```python
from build123d import *

# Parameters (mm, degrees)
SKETCH1_R        = 8
EXTRUSION1_DEPTH = 400
SKETCH2_R        = 8
EXTRUSION2_DEPTH = 50
EXTRUSION3_START = 50
SKETCH3_R        = 8
EXTRUSION3_DEPTH = 50
SKETCH4_R        = 8
SKETCH4_R_2      = 6
THREAD1_DEPTH    = 14
SKETCH5_R        = 8
SKETCH5_R_2      = 6.05
EXTRUSION5_DEPTH = 25
SKETCH6_R        = 5
EXTRUSION6_DEPTH = 15
EXTRUSION7_START = -27.101
SKETCH7_R        = 8
EXTRUSION7_DEPTH = 27.101
EXTRUSION8_START = 12
SKETCH8_R        = 5
EXTRUSION8_DEPTH = 12


with BuildPart() as part:
    # Sketch1 → Extrusion1 (new body)
    with BuildSketch(Plane(origin=(0, 0, 0), x_dir=(-1, 0, 0), z_dir=(0, 1, 0))):
        with Locations(Location((0, 0, 0), (0, 0, 90))):
            Circle(SKETCH1_R)
    extrude(amount=EXTRUSION1_DEPTH)

    # Sketch2 → Extrusion2 (cut)
    with BuildSketch(Plane.XZ):
        with Locations(Location((0, 0, 0), (0, 0, 270))):
            Circle(SKETCH2_R)
    extrude(amount=-EXTRUSION2_DEPTH, mode=Mode.SUBTRACT)

    # Sketch3 → Extrusion3 (add)
    with BuildSketch(Plane.XZ.offset(-50).offset(EXTRUSION3_START)):
        with Locations(Location((0, 0, 0), (0, 0, 270))):
            Circle(SKETCH3_R)
    extrude(amount=-EXTRUSION3_DEPTH)

    # Sketch4 → Thread1 (cut)
    with BuildSketch(Plane.XZ):
        with Locations(Location((0, 0, 0), (0, 0, 270))):
            Circle(SKETCH4_R)
        with Locations(Location((0, 0, 0), (0, 0, 270))):
            Circle(SKETCH4_R_2, mode=Mode.SUBTRACT)
    extrude(amount=-THREAD1_DEPTH, mode=Mode.SUBTRACT)

    # Sketch5 → Extrusion5 (cut)
    with BuildSketch(Plane.XZ.offset(-14)):
        with Locations(Location((0, 0, 0), (0, 0, 270))):
            Circle(SKETCH5_R)
        with Locations(Location((0, 0, 0), (0, 0, 270))):
            Circle(SKETCH5_R_2, mode=Mode.SUBTRACT)
    extrude(amount=-EXTRUSION5_DEPTH, mode=Mode.SUBTRACT)

    # Sketch6 → Extrusion6 (add)
    with BuildSketch(Plane.XZ):
        with Locations(Location((0, 0, 0), (0, 0, 270))):
            Circle(SKETCH6_R)
    extrude(amount=EXTRUSION6_DEPTH)

    # Sketch7 → Extrusion7 (cut)
    with BuildSketch(Plane(origin=(0, 400, 0), x_dir=(-1, 0, 0), z_dir=(0, 1, 0)).offset(EXTRUSION7_START)):
        with Locations(Location((0, 0, 0), (0, 0, 270))):
            Circle(SKETCH7_R)
    extrude(amount=EXTRUSION7_DEPTH, mode=Mode.SUBTRACT)

    # Sketch8 → Extrusion8 (add)
    with BuildSketch(Plane(origin=(0, 372.899, 0), x_dir=(-1, 0, 0), z_dir=(0, 1, 0)).offset(EXTRUSION8_START)):
        with Locations(Location((0, 0, 0), (0, 0, 270))):
            Circle(SKETCH8_R)
    extrude(amount=-EXTRUSION8_DEPTH)


solid = part.part
```
Check sheet for the modelled part. Datum: model origin and axes. Units: mm. A direction names the side the tool comes from. Coordinates: 2 decimals unless noted, no trailing zeros. Order: outer loops, then holes, each group sorted by start corner. A loop starts at its lowest first (then second) coordinate and runs counter-clockwise, first axis right, second up. Notation, with made-up numbers: (34, 64) -> (62, 64) arc R20 ccw to (62, 77) -> close; hole circle Ø4 at (-6, 62.25). An arc over 180 degrees is marked (long way). Write each question's results on one line, items separated by ' | '. Start each with the question number.
1) Depth check by flat-ended pin: pin 1 (1 mm diameter, centred on y = 310.5, z = -6.5, fed in from +X); pin 2 (3 mm diameter, centred on x = 6, z = 4.5, fed in from +Y); pin 3 (2 mm diameter, centred on x = -3.5, y = 45, fed in from +Z); pin 4 (1.5 mm diameter, centred on x = 2.5, z = -4.5, fed in from -Y). Enter the tip coordinate at first touch or a pass-through.
2) Section check C-C (y = 67.5). Enter the section's corners in (x, z).
3) Material ranges on line 1 along X through (y, z) = (357, 0.5); line 2 along Z through (x, y) = (0.75, 297); line 3 along Y through (x, z) = (-1.75, -7), recorded low to high.
4) Set-up check for faces 1 (the face through (0, 384.899, 0)), 2 (the face through (4, 0, 4)), 3 (the face through (5.2, 372.899, 0.1)): record each of +Z, -Z, +X, -X, +Y, -Y from which the full face is reachable in a straight line by a thin tool's end or side.
5) Section check A-A (x = 0). Enter the section's corners in (y, z), and give its area (3 significant figures).
6) Section check B-B (z = 0). Enter the section's corners in (x, y).
Checked values:
1) pin 1: x = 5.29 | pin 2: y = 372.9 | pin 3: z = 7.6 | pin 4: y = -15
2) outline: circle Ø16 at (0, 0)
3) line 1: -7.98 to 7.98 | line 2: -7.96 to 7.96 | line 3: 39 to 372.9
4) face 1: +Z, -Z, +X, -X, +Y | face 2: -Y | face 3: +Y
5) outline: (-15, -5) -> (0, -5) -> (0, -6) -> (14, -6) -> (14, -6.05) -> (39, -6.05) -> (39, -8) -> (372.9, -8) -> (372.9, -5) -> (384.9, -5) -> (384.9, 5) -> (372.9, 5) -> (372.9, 8) -> (39, 8) -> (39, 6.05) -> (14, 6.05) -> (14, 6) -> (0, 6) -> (0, 5) -> (-15, 5) -> close | area: 6,080 mm²
6) outline: (-8, 39) -> (-6.05, 39) -> (-6.05, 14) -> (-6, 14) -> (-6, 0) -> (-5, 0) -> (-5, -15) -> (5, -15) -> (5, 0) -> (6, 0) -> (6, 14) -> (6.05, 14) -> (6.05, 39) -> (8, 39) -> (8, 372.9) -> (5, 372.9) -> (5, 384.9) -> (-5, 384.9) -> (-5, 372.9) -> (-8, 372.9) -> close
